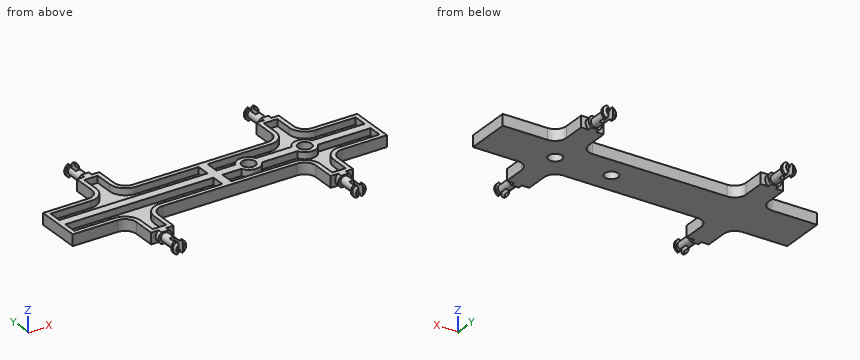
```python
from build123d import *

# Parameters (mm, degrees)
F1_DEPTH  = 2.5
F2_T      = -2
F5_SIZE   = 1
F6_W      = 101.6216283701
F6_H      = 5
F7_DEPTH  = 37.501
F8_W      = 2
F8_H      = 12.9450548419
F9_DEPTH  = 6
F12_R     = 5
F13_DEPTH = 5
F15_D     = 6
F19_ANGLE = 90
F21_ANGLE = 180


with BuildPart() as f1:
    # F0 (on Front) → F1 (new body, symmetric)
    with BuildSketch(Plane.XZ):
        with BuildLine():
            Line((-42.8484990943, 10), (-42.8484990943, 0))
            Line((-42.8484990943, 0), (27.1515009057, 0))
            Line((27.1515009057, 0), (27.1515009057, 10))
            Line((27.1515009057, 10), (7.1515009057, 10))
            ThreePointArc((7.1515009057, 10), (3.6159669998, 11.4644660941), (2.1515009057, 15))
            Line((2.1515009057, 15), (2.1515009057, 25))
            Line((2.1515009057, 25), (-7.8484990943, 25))
            Line((-7.8484990943, 25), (-7.8484990943, 15))
            ThreePointArc((-7.8484990943, 15), (-9.3129651884, 11.4644660941), (-12.8484990943, 10))
            Line((-12.8484990943, 10), (-42.8484990943, 10))
        make_face()
    extrude(amount=F1_DEPTH, both=True)

    # F2
    f2_openings = [f1.faces().sort_by_distance(p)[0] for p in [
        (-6.914814, -2.5, 7.254637),
    ]]
    offset(amount=F2_T, openings=f2_openings)

    # F3 (on Front) → F4 (revolve)
    with BuildSketch(Plane.XZ):
        Polygon((-2.8484990943, 37.5), (-5.8484990943, 37.5), (-5.8484990943, 35.5), (-4.8484990943, 35.5), (-4.8484990943, 27), (-5.8484990943, 27), (-5.8484990943, 25), (-2.8484990943, 25), align=None)
    revolve(axis=Axis((-2.8484990943, 0, 31.25), (0, 0, -1)))

    # F5
    f5_edges = [f1.edges().sort_by_distance(p)[0] for p in [
        (0.151501, 0, 37.5),
    ]]
    chamfer(f5_edges, length=F5_SIZE)

    # F6 (on face) → F7 (intersect, through all)
    with BuildSketch(Plane.XY.offset(37.5)):
        with Locations((-4.4455640018, 0)):
            Rectangle(F6_W, F6_H)
    extrude(amount=-F7_DEPTH, mode=Mode.INTERSECT)

    # F8 (on face) → F9 (cut)
    with BuildSketch(Plane.XY.offset(37.5)):
        with Locations((-2.8484990943, -0.3656100016)):
            Rectangle(F8_W, F8_H)
    extrude(amount=-F9_DEPTH, mode=Mode.SUBTRACT)

    # F10: F1 across plane


with BuildPart() as f1_1:
    add(f1.part)
    add(f1.part.mirror(Plane.XY))

    # F11: F1 across face


with BuildPart() as f1_2:
    add(f1_1.part)
    add(f1_1.part.mirror(Plane(origin=(-42.8484990943, 0, 0), x_dir=(0, -1, 0), z_dir=(-1, 0, 0))))

    # F12 (on face) → F13 (join, through all)
    with BuildSketch(Plane.XZ.offset(2.5)):
        with Locations((-2.8484990943, 0)):
            Circle(F12_R)
        with Locations((-27.8484990943, 0)):
            Circle(F12_R)
    extrude(amount=-F13_DEPTH)

    # F15 (through all)
    with Locations(Plane.XZ.offset(2.5)):
        with Locations((-27.8484990943, 0), (-2.8484990943, 0)):
            Hole(F15_D / 2)


with BuildPart() as f1_3:
    # F16: moved
    add(f1_2.part.moved(Location((40, 0, 0))))


with BuildPart() as f1_4:
    # F17: moved
    add(f1_3.part.moved(Location((5, 0, 0))))


with BuildPart() as f1_5:
    # F18: moved
    add(f1_4.part.moved(Location((-2.5, 0, 0))))


with BuildPart() as f1_6:
    # F19: moved
    add(f1_5.part.rotate(Axis((59.6515009057, 2.5, 10), (1, 0, 0)), F19_ANGLE))


with BuildPart() as f1_7:
    # F20: moved
    add(f1_6.part.moved(Location((0, 0, -7.5))))


with BuildPart() as f1_8:
    # F21: moved
    add(f1_7.part.rotate(Axis((-60.3484990943, 2.5, -2.5), (-1, 0, 0)), F21_ANGLE))


with BuildPart() as f1_9:
    # F22: moved
    add(f1_8.part.moved(Location((0, 0, 5))))


solid = f1_9.part
```
The listing builds one solid part. Answer for the finished solid, in the listing's coordinates (mm). Coordinates: 2 decimals unless noted, no trailing zeros. Write each loop counter-clockwise with the first axis right and the second up, starting at its lowest first coordinate (ties: lowest second). Pieces come first, ordered by that corner, then holes. Notation, with made-up numbers: (63, 54) - (99, 54) arc R25 ccw to (99, 67) - close; hole circle Ø10 at (55, 78.25). An arc over 180 degrees is marked (long way). Return JSON: item names as keys, results as strings. Group by question number.
1. A cutting plane is placed at B-B, the plane y = -7.5. Determine the outline of the cut face in (x, z).
2. Straight lines are drawn through the part: L1, parallel to Y at x = -20, z = 2.1; L2, parallel to X at y = 0, z = 0.5; L3, parallel to X at y = -23, z = 1.1. For each, find the intervals that lie inside material, in ascending order.
3. A cutting plane is placed at D-D, the plane y = -36. Determine the outline of the cut face in (x, z), plus the area to 3 significant figures.
4. A cutting plane is placed at A-A, the plane y = 9.5. Determine the outline of the cut face in (x, z).
5. Given pin 1 (0.6 mm diameter, centred on x = 40, z = -0.5, fed in from -Y); pin 2 (2.5 mm diameter, centred on x = 1.5, z = 0, fed in from -Y); pin 3 (0.6 mm diameter, centred on x = 42, z = 0, fed in from +Y), each flat-ended and moving along its own axis, determine where each tip first touches the part or whether it passes through.
6. A cutting plane is placed at C-C, the plane x = -12.5. Determine the outline of the cut face in (y, z).
Ans:
{
 "1": {"outline": "(-70.35, -2.5) - (11.65, -2.5) - (11.65, 2.5) - (-70.35, 2.5) - close; (17.65, -2.5) - (36.65, -2.5) - (36.65, 2.5) - (17.65, 2.5) - close; (42.65, -2.5) - (69.65, -2.5) - (69.65, 2.5) - (42.65, 2.5) - close"},
 "2": {"L1": "-17.5 to -15.5, -9.5 to -5.5, 0.5 to 2.5", "L2": "-70.35 to -68.35, -2.35 to 1.65, 67.65 to 69.65", "L3": "-45.35 to -43.35, -37.35 to -35.35, 34.65 to 36.65, 42.65 to 44.65"},
 "3": {"outline": "circle Ø4 at (-40.35, 0); circle Ø4 at (39.65, 0)", "area": "25.1 mm²"},
 "4": {"outline": "(-45.35, -2.5) - (-35.35, -2.5) - (-35.35, 2.5) - (-37.35, 2.5) - (-37.35, -0.5) - (-43.35, -0.5) - (-43.35, 2.5) - (-45.35, 2.5) - close; (34.65, -2.5) - (44.65, -2.5) - (44.65, 2.5) - (42.65, 2.5) - (42.65, -0.5) - (36.65, -0.5) - (36.65, 2.5) - (34.65, 2.5) - close"},
 "5": {"pin 1": "y = -39", "pin 2": "y = -17.5", "pin 3": "y = 29.95"},
 "6": {"outline": "(-17.5, -2.5) - (2.5, -2.5) - (2.5, 2.5) - (0.5, 2.5) - (0.5, -0.5) - (-5.5, -0.5) - (-5.5, 2.5) - (-9.5, 2.5) - (-9.5, -0.5) - (-15.5, -0.5) - (-15.5, 2.5) - (-17.5, 2.5) - close"}
}
